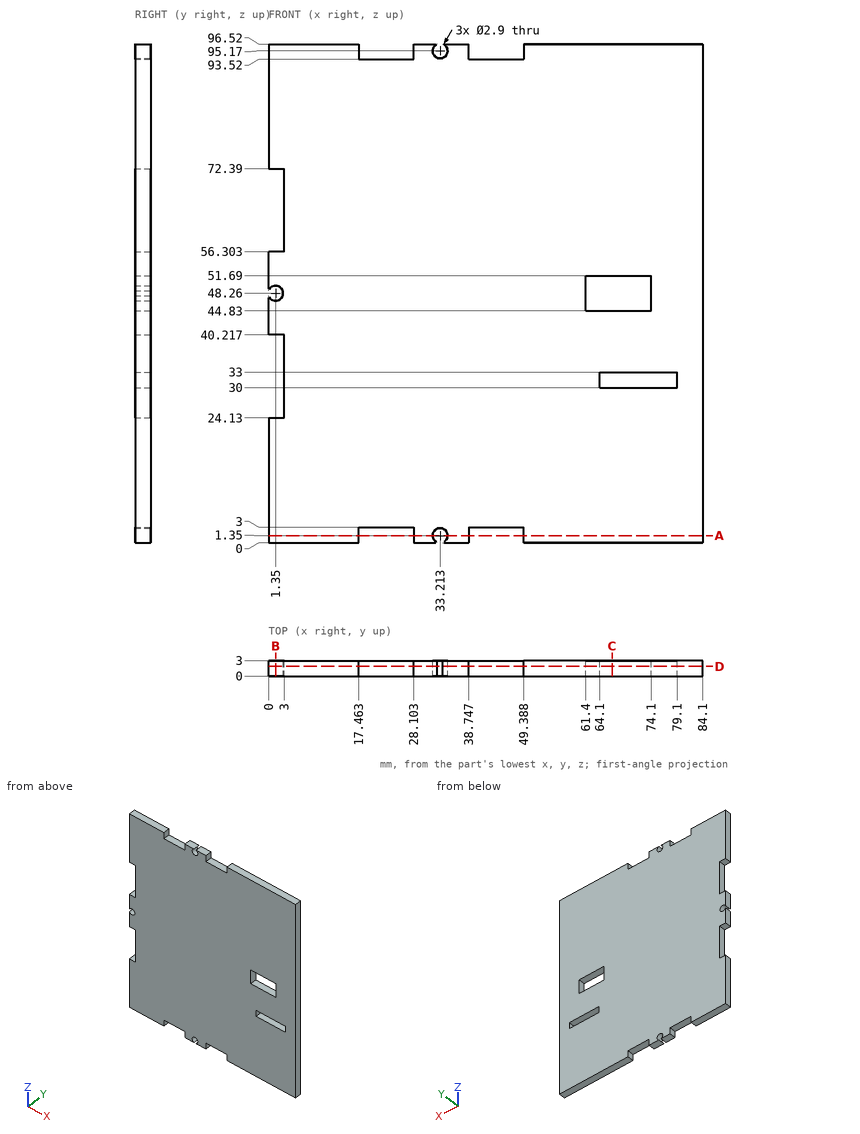
The figure shows three views and two pictorial views of one solid part (mm, origin at its lowest corner). Answer the questions. Give positions to 0.01 mm unless a question says otherwise; leave off trailing zeros. Write each loop counter-clockwise with the first axis right and the second up, starting at its lowest first coordinate (ties: lowest second). Pieces come first, ordered by that corner, then holes.
Q1. Given pin 1 (0.9 mm diameter, centred on x = 44.5, y = 1, fed in from -Z); pin 2 (1.5 mm diameter, centred on y = 1, z = 65.5, fed in from -X), each flat-ended and moving along its own axis, determine where each tip first touches the part or whether it passes through.
Answer:
pin 1: stops at z = 3
pin 2: stops at x = 3
Q2. The part is cut by section A-A on z = 1.35. Give the vertices of the cut face in (x, y), and give its area (3 significant figures).
Answer:
outline: (0, 0) - (17.46, 0) - (17.46, 3) - (0, 3) - close; (28.1, 0) - (31.76, 0) - (31.76, 3) - (28.1, 3) - close; (34.66, 0) - (38.75, 0) - (38.75, 3) - (34.66, 3) - close; (49.39, 0) - (84.1, 0) - (84.1, 3) - (49.39, 3) - close
area: 180 mm2
Q3. The part is cut by section D-D on y = 1.85. State how many separate pieces and enclosed holes the cut face has, and give its area (3 significant figures).
Answer:
separate pieces: 1
enclosed holes: 2
area: 7,740 mm2
Q4. Straight lines are drawn through the part: L1, parallel to X at y = 1.75, z = 1.35; L2, parallel to X at y = 1.45, z = 64.5; L3, parallel to Z at x = 44.5, y = 0.95. For each, find the intervals that lie inside material, in ascending order.
Answer:
L1: x = 0 to 17.46, 28.1 to 31.76, 34.66 to 38.75, 49.39 to 84.1
L2: x = 3 to 84.1
L3: z = 3 to 93.52
Q5. The part is cut by section C-C on x = 66.5. Give the vertices of the cut face in (y, z).
Answer:
outline: (0, 0) - (3, 0) - (3, 30) - (0, 30) - close; (0, 33) - (3, 33) - (3, 44.83) - (0, 44.83) - close; (0, 51.69) - (3, 51.69) - (3, 96.52) - (0, 96.52) - close
Q6. The part is cut by section B-B on x = 1.35. Give the vertices of the cut face in (y, z), and give its area (3 significant figures).
Answer:
outline: (0, 0) - (3, 0) - (3, 24.13) - (0, 24.13) - close; (0, 40.22) - (3, 40.22) - (3, 46.81) - (0, 46.81) - close; (0, 49.71) - (3, 49.71) - (3, 56.3) - (0, 56.3) - close; (0, 72.39) - (3, 72.39) - (3, 96.52) - (0, 96.52) - close
area: 184 mm2
